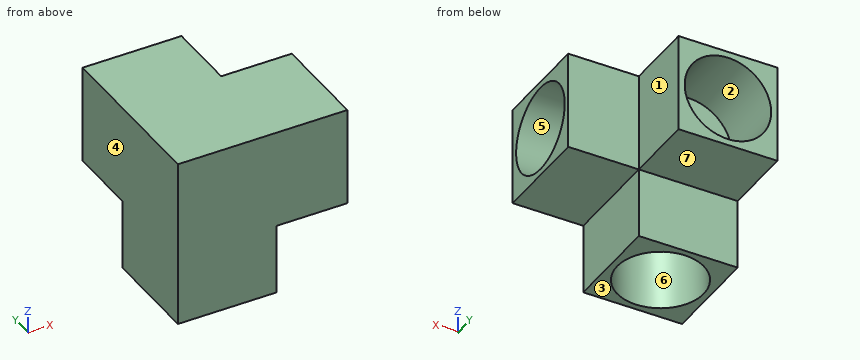
from build123d import *

# Parameters (mm, degrees)
F0_W      = 28
F0_H      = 28
F1_DEPTH  = 48
F2_W      = 28
F2_H      = 28
F3_DEPTH  = 48
F4_W      = 28
F4_H      = 28
F5_DEPTH  = 48
F6_R      = 12.25
F7_DEPTH  = 20
F8_R      = 12.25
F9_DEPTH  = 20
F10_R     = 12.25
F11_DEPTH = 20


with BuildPart() as f1:
    # F0 (on Right) → F1 (new body)
    with BuildSketch(Plane.YZ):
        Rectangle(F0_W, F0_H)
    extrude(amount=F1_DEPTH)

    # F2 (on face) → F3 (join)
    with BuildSketch(Plane.XZ.offset(14)):
        with Locations((14, 0)):
            Rectangle(F2_W, F2_H)
    extrude(amount=-F3_DEPTH)

    # F4 (on face) → F5 (join)
    with BuildSketch(Plane.XY.offset(14)):
        with Locations((14, 0)):
            Rectangle(F4_W, F4_H)
    extrude(amount=-F5_DEPTH)

    # F6 (on face) → F7 (cut)
    with BuildSketch(Plane.YZ.offset(48)):
        Circle(F6_R)
    extrude(amount=-F7_DEPTH, mode=Mode.SUBTRACT)

    # F8 (on face) → F9 (cut)
    with BuildSketch(Plane(origin=(0, 34, 0), x_dir=(-1, 0, 0), z_dir=(0, 1, 0))):
        with Locations((-14, 0)):
            Circle(F8_R)
    extrude(amount=-F9_DEPTH, mode=Mode.SUBTRACT)

    # F10 (on face) → F11 (cut)
    with BuildSketch(Plane(origin=(0, 0, -34), x_dir=(1, 0, 0), z_dir=(0, 0, -1))):
        with Locations((14, 0)):
            Circle(F10_R)
    extrude(amount=-F11_DEPTH, mode=Mode.SUBTRACT)


solid = f1.part
Here's how the part is built. I have some questions about the finished solid (model axes, mm). Face numbers are marked on the shaded views. A direction names the side the tool comes from. Coordinates: 2 decimals unless noted, no trailing zeros. Loops run counter-clockwise (first coordinate to the right, second up) from the corner with the lowest first, then second, coordinate; pieces in that order, holes last. Notation, with made-up numbers: (-5, 54.25) -> (4, 54.25) arc R15 cw to (4, 68.25) -> close; hole circle Ø4 at (-14.5, 21). An arc over 180 degrees is marked (long way). Use one line per item in the form item = value. Start each with the question number.
(1) On a 3-axis mill with a long thin cutter (end or side, diameter ignored), from which of +Z, -Z, +X, -X, +Y, -Y can I reach the whole of each face in a straight line? I mean the marked faces 5, 6 and 7. Say none if no direction works.
(2) If we section it at C-C (z = 0): Please give me the cut outline in (x, y), then the cut area to 3 significant figures.
(3) We'd pull the mould along X, two halves only. Please class the marked faces 1, 2, 3 and 4: pulls with the +X half, pulls with the -X half, needs draft (parallel to the pull), parting line crosses it, or undercut.
(4) If we section it at D-D (y = 0): Please give me the cut outline in (x, z), then the cut area to 3 significant figures.
(5) If we section it at A-A (z = -20): Please give me the cut outline in (x, y).
(6) Please list where these lines run through material, in increasing order: line 1 along Z through (x, y) = (43, 0); line 2 along X through (y, z) = (0, -27).
(7) Will these pins go through, and if not, where does the flat tip stop? pin 1 (7.5 mm diameter, centred on y = 5, z = 5.5, fed in from +X); pin 2 (8 mm diameter, centred on x = 38.5, z = -4, fed in from +Y); pin 3 (22 mm diameter, centred on x = 13.5, y = 26, fed in from -Z).
(8) If we section it at B-B (x = 38.5): Please give me the cut outline in (y, z), then the cut area to 3 significant figures.
Verdict:
q1.face_5 = +X
q1.face_6 = -Z
q1.face_7 = -Z, +X, -X, +Y
q2.outline = (0, -14) -> (48, -14) -> (48, -12.25) -> (28, -12.25) -> (28, 12.25) -> (48, 12.25) -> (48, 14) -> (28, 14) -> (28, 34) -> (26.25, 34) -> (26.25, 14) -> (1.75, 14) -> (1.75, 34) -> (0, 34) -> close
q2.area = 924 mm²
q3.face_1 = pulls with the +X half
q3.face_2 = undercut
q3.face_3 = needs draft
q3.face_4 = pulls with the -X half
q4.outline = (0, -34) -> (1.75, -34) -> (1.75, -14) -> (26.25, -14) -> (26.25, -34) -> (28, -34) -> (28, -14) -> (48, -14) -> (48, -12.25) -> (28, -12.25) -> (28, 12.25) -> (48, 12.25) -> (48, 14) -> (0, 14) -> close
q4.area = 924 mm²
q5.outline = (0, -14) -> (28, -14) -> (28, 14) -> (0, 14) -> close; hole circle Ø24.5 at (14, 0)
q6.line_1 = -14 to -12.25, 12.25 to 14
q6.line_2 = 0 to 1.75, 26.25 to 28
q7.pin_1 = 28
q7.pin_2 = 14
q7.pin_3 = -14
q8.outline = (-14, -14) -> (14, -14) -> (14, 14) -> (-14, 14) -> close; hole circle Ø24.5 at (0, 0)
q8.area = 313 mm²
